from build123d import *

# Parameters (mm, degrees)
SKETCH1_R           = 2.5
SKETCH1_R_2         = 1.55
SKETCH1_W           = 4
SKETCH1_H           = 10.16
BOSS_EXTRUDE1_DEPTH = 4


with BuildPart() as part:
    # Sketch1 → Boss-Extrude1 (new body)
    with BuildSketch(Plane.XY):
        with BuildLine():
            Line((0, 10.16), (4, 10.16))
            Line((4, 10.16), (4, 13.97))
            Line((4, 13.97), (5.81, 13.97))
            ThreePointArc((5.81, 13.97), (8.504076836, 12.854076836), (9.62, 10.16))
            Line((9.62, 10.16), (9.62, -70.001621467))
            ThreePointArc((9.62, -70.001621467), (9.700768986, -71.10814563), (9.941363707, -72.191212355))
            Line((9.941363707, -72.191212355), (13.108636293, -82.748787645))
            ThreePointArc((13.108636293, -82.748787645), (13.349231014, -83.83185437), (13.43, -84.938378533))
            Line((13.43, -84.938378533), (13.43, -97.79))
            ThreePointArc((13.43, -97.79), (11.198153673, -103.178153673), (5.81, -105.41))
            Line((5.81, -105.41), (-1.81, -105.41))
            ThreePointArc((-1.81, -105.41), (-7.198153673, -103.178153673), (-9.43, -97.79))
            Line((-9.43, -97.79), (-9.43, -84.938378533))
            ThreePointArc((-9.43, -84.938378533), (-9.349231014, -83.83185437), (-9.108636293, -82.748787645))
            Line((-9.108636293, -82.748787645), (-5.941363707, -72.191212355))
            ThreePointArc((-5.941363707, -72.191212355), (-5.700768986, -71.10814563), (-5.62, -70.001621467))
            Line((-5.62, -70.001621467), (-5.62, 10.16))
            ThreePointArc((-5.62, 10.16), (-4.504076836, 12.854076836), (-1.81, 13.97))
            Line((-1.81, 13.97), (0, 13.97))
            Line((0, 13.97), (0, 10.16))
        make_face()
        with Locations((2, -93.98)):
            Circle(SKETCH1_R, mode=Mode.SUBTRACT)
        with Locations((7.656854249, -88.323145751)):
            Circle(SKETCH1_R_2, mode=Mode.SUBTRACT)
        with Locations((-3.656854249, -88.323145751)):
            Circle(SKETCH1_R_2, mode=Mode.SUBTRACT)
        with Locations((-3.656854249, -99.636854249)):
            Circle(SKETCH1_R_2, mode=Mode.SUBTRACT)
        with Locations((7.656854249, -99.636854249)):
            Circle(SKETCH1_R_2, mode=Mode.SUBTRACT)
        with Locations((2, -5.08)):
            Rectangle(SKETCH1_W, SKETCH1_H, mode=Mode.SUBTRACT)
        with Locations((2, -25.4)):
            Rectangle(SKETCH1_W, SKETCH1_H, mode=Mode.SUBTRACT)
    extrude(amount=BOSS_EXTRUDE1_DEPTH)


solid = part.part
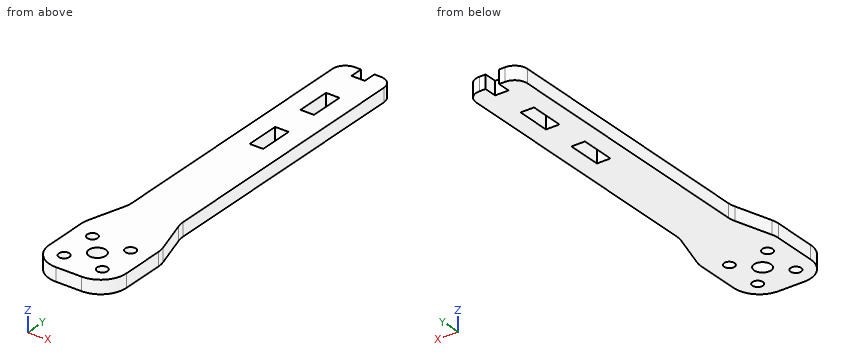
Geometry: final body of the model. Coordinates: model frame, mm. Give positions to 0.01 mm unless a question says otherwise; leave off trailing zeros. Write each loop counter-clockwise with the first axis right and the second up, starting at its lowest first coordinate (ties: lowest second). Pieces come first, ordered by that corner, then holes. Notation, with made-up numbers: (39, -33) - (86, -33) arc R30 cw to (86, 3) - close; hole circle Ø6 at (22, -33.5). An arc over 180 degrees is marked (long way). Return JSON: item names as keys, results as strings. Group by question number.
1) Line query: line 1 (Y direction, x = 2, z = 0.85); line 2 (X direction, y = -8.5, z = 2.05); line 3 (Y direction, x = -2.5, z = 2.7). Output: solid intervals per line, ascending.
2) Section D-D on z = 3.15. State how many separate pieces and enclosed holes the cut face has, plus the area to 3 significant figures.
3) First-contact query: P1, Ø3, axis at x = -3.66, y = -88.32, coming from the -Z side; P2, Ø2, axis at y = -6, z = 1.5, coming from the -X side; P3, Ø1.2, axis at x = 1.5, z = 3, coming from the +Y side; P4, Ø1.5, axis at y = -25, z = 2.5, coming from the +X side. Flat tips, straight axial feed; report the tip coordinate or a pass-through.
4) Section C-C on y = -7. Return the cut outline in (x, z).
5) Section B-B on x = 2. Return the cut outline in (y, z).
6) Section A-A on y = -93.98. Return the cut outline in (x, z), plus the area to 3 significant figures.
Filled in:
{
 "1": {"line 1": "y = -105.41 to -96.48, -91.48 to -30.48, -20.32 to -10.16, 0 to 10.16", "line 2": "x = -5.62 to 0, 4 to 9.62", "line 3": "y = -105.38 to -100.67, -98.61 to -89.35, -87.29 to 13.91"},
 "2": {"separate pieces": "1", "enclosed holes": "7", "area": "1,850 mm^2"},
 "3": {"P1": "passes through", "P2": "stops at x = -5.62", "P3": "stops at y = 10.16", "P4": "stops at x = 9.62"},
 "4": {"outline": "(-5.62, 0) - (0, 0) - (0, 4) - (-5.62, 4) - close; (4, 0) - (9.62, 0) - (9.62, 4) - (4, 4) - close"},
 "5": {"outline": "(-105.41, 0) - (-96.48, 0) - (-96.48, 4) - (-105.41, 4) - close; (-91.48, 0) - (-30.48, 0) - (-30.48, 4) - (-91.48, 4) - close; (-20.32, 0) - (-10.16, 0) - (-10.16, 4) - (-20.32, 4) - close; (0, 0) - (10.16, 0) - (10.16, 4) - (0, 4) - close"},
 "6": {"outline": "(-9.43, 0) - (-0.5, 0) - (-0.5, 4) - (-9.43, 4) - close; (4.5, 0) - (13.43, 0) - (13.43, 4) - (4.5, 4) - close", "area": "71.4 mm^2"}
}
